For this review, take the finished solid that the model builds, in its own axes (mm). Round coordinates to 2 decimals unless told otherwise and drop trailing zeros. Loops run counter-clockwise (first coordinate to the right, second up) from the corner with the lowest first, then second, coordinate; pieces in that order, holes last.
1) Take a section at A-A (y = 2.5). Give the number of separate pieces and of enclosed holes in the cut face, then the cut area to 3 significant figures.
2) Take a section at B-B (z = 106). State the section outline as (x, y) points, then the cut area to 3 significant figures.
3) Insertion check: pin 1 (1.5 mm diameter, centred on y = 1, z = -52, fed in from -X); pin 2 (0.9 mm diameter, centred on y = 1.5, z = -148, fed in from -X); pin 3 (0.9 mm diameter, centred on x = -98.5, y = 1.5, fed in from +Z). Each pin has a flat end and moves straight along its axis. Give the tip position at first contact, or say it passes through.
4) Wall thickness on L1, parallel to X at y = 2.05, z = 68; L2, parallel to Z at x = 0, y = 1.8; L3, parallel to X at y = 0.95, z = -54.5: over which ranges is each line inside the solid? List them lowest first.
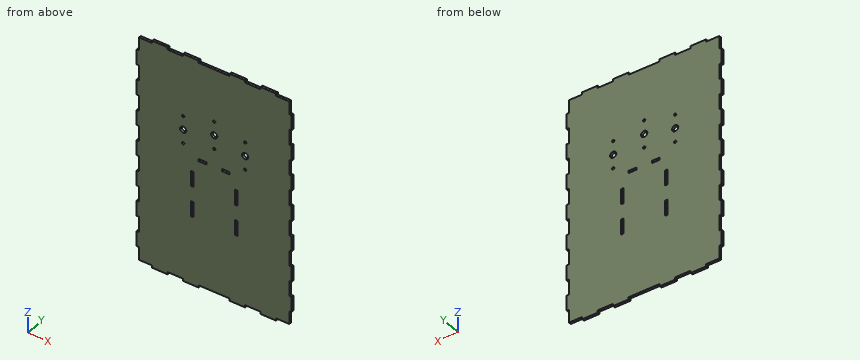
```python
from build123d import *

# Parameters (mm, degrees)
SKETCH1_W           = 200
SKETCH1_H           = 300
BOSS_EXTRUDE1_DEPTH = 3
SKETCH2_W           = 3
SKETCH2_H           = 20
SKETCH2_W_2         = 10
SKETCH2_H_2         = 3
CUT_EXTRUDE1_DEPTH  = 3
SKETCH3_W           = 3
SKETCH3_H           = 20
SKETCH3_W_2         = 20
SKETCH3_H_2         = 3
SKETCH3_W_3         = 40
CUT_EXTRUDE2_DEPTH  = 3
SKETCH4_R           = 4
SKETCH4_R_2         = 1.5
CUT_EXTRUDE3_DEPTH  = 3


with BuildPart() as part:
    # Sketch1 → Boss-Extrude1 (new body)
    with BuildSketch(Plane(origin=(0, 0, 0), x_dir=(1, 0, 0), z_dir=(0, 1, 0))):
        Rectangle(SKETCH1_W, SKETCH1_H)
    extrude(amount=BOSS_EXTRUDE1_DEPTH)

    # Sketch2 → Cut-Extrude1 (cut)
    with BuildSketch(Plane(origin=(0, 3, 0), x_dir=(1, 0, 0), z_dir=(0, 1, 0))):
        with Locations((-28.5, 10)):
            Rectangle(SKETCH2_W, SKETCH2_H)
        with Locations((28.5, 10)):
            Rectangle(SKETCH2_W, SKETCH2_H)
        with Locations((15, -18.5)):
            Rectangle(SKETCH2_W_2, SKETCH2_H_2)
        with Locations((28.5, 50)):
            Rectangle(SKETCH2_W, SKETCH2_H)
        with Locations((-28.5, 50)):
            Rectangle(SKETCH2_W, SKETCH2_H)
        with Locations((-15, -18.5)):
            Rectangle(SKETCH2_W_2, SKETCH2_H_2)
    extrude(amount=-CUT_EXTRUDE1_DEPTH, mode=Mode.SUBTRACT)

    # Sketch3 → Cut-Extrude2 (cut)
    with BuildSketch(Plane(origin=(0, 3, 0), x_dir=(1, 0, 0), z_dir=(0, 1, 0))):
        Polygon((100, 130), (97, 130), (97, 147), (80, 147), (80, 150), (100, 150), align=None)
        with Locations((98.5, 100)):
            Rectangle(SKETCH3_W, SKETCH3_H)
        with Locations((98.5, 60)):
            Rectangle(SKETCH3_W, SKETCH3_H)
        Polygon((-100, 150), (-100, 130), (-97, 130), (-97, 147), (-80, 147), (-80, 150), align=None)
        Polygon((-100, -150), (-80, -150), (-80, -147), (-97, -147), (-97, -130), (-100, -130), align=None)
        Polygon((100, -150), (100, -130), (97, -130), (97, -147), (80, -147), (80, -150), align=None)
        with Locations((98.5, 20)):
            Rectangle(SKETCH3_W, SKETCH3_H)
        with Locations((98.5, -20)):
            Rectangle(SKETCH3_W, SKETCH3_H)
        with Locations((98.5, -60)):
            Rectangle(SKETCH3_W, SKETCH3_H)
        with Locations((98.5, -100)):
            Rectangle(SKETCH3_W, SKETCH3_H)
        with Locations((-98.5, 100)):
            Rectangle(SKETCH3_W, SKETCH3_H)
        with Locations((-98.5, 60)):
            Rectangle(SKETCH3_W, SKETCH3_H)
        with Locations((-98.5, 20)):
            Rectangle(SKETCH3_W, SKETCH3_H)
        with Locations((-98.5, -20)):
            Rectangle(SKETCH3_W, SKETCH3_H)
        with Locations((-98.5, -60)):
            Rectangle(SKETCH3_W, SKETCH3_H)
        with Locations((-98.5, -100)):
            Rectangle(SKETCH3_W, SKETCH3_H)
        with Locations((-50, 148.5)):
            Rectangle(SKETCH3_W_2, SKETCH3_H_2)
        with Locations((0, 148.5)):
            Rectangle(SKETCH3_W_3, SKETCH3_H_2)
        with Locations((50, 148.5)):
            Rectangle(SKETCH3_W_2, SKETCH3_H_2)
        with Locations((50, -148.5)):
            Rectangle(SKETCH3_W_2, SKETCH3_H_2)
        with Locations((0, -148.5)):
            Rectangle(SKETCH3_W_3, SKETCH3_H_2)
        with Locations((-50, -148.5)):
            Rectangle(SKETCH3_W_2, SKETCH3_H_2)
    extrude(amount=-CUT_EXTRUDE2_DEPTH, mode=Mode.SUBTRACT)

    # Sketch4 → Cut-Extrude3 (cut)
    with BuildSketch(Plane(origin=(0, 3, 0), x_dir=(1, 0, 0), z_dir=(0, 1, 0))):
        with Locations((0, -60)):
            Circle(SKETCH4_R)
        with Locations((40, -50)):
            Circle(SKETCH4_R)
        with Locations((-40, -50)):
            Circle(SKETCH4_R)
        with Locations((40, -32)):
            Circle(SKETCH4_R_2)
        with Locations((40, -68)):
            Circle(SKETCH4_R_2)
        with Locations((0, -42)):
            Circle(SKETCH4_R_2)
        with Locations((0, -78)):
            Circle(SKETCH4_R_2)
        with Locations((-40, -32)):
            Circle(SKETCH4_R_2)
        with Locations((-40, -68)):
            Circle(SKETCH4_R_2)
    extrude(amount=-CUT_EXTRUDE3_DEPTH, mode=Mode.SUBTRACT)


solid = part.part
```
Response:
1. separate pieces: 1
1. enclosed holes: 15
1. area: 57,900 mm2
2. outline: (-97, 0) - (97, 0) - (97, 3) - (-97, 3) - close
2. area: 582 mm2
3. pin 1: stops at x = -97
3. pin 2: stops at x = -80
3. pin 3: stops at z = 130
4. L1: x = -97 to -41.5, -38.5 to 38.5, 41.5 to 97
4. L2: z = -147 to 40.5, 43.5 to 56, 64 to 76.5, 79.5 to 147
4. L3: x = -97 to -30, -27 to 27, 30 to 97
